Check sheet for the drawn part. Datum: minimum x, y, z corner. Units: mm. A direction names the side the tool comes from. Coordinates: 2 decimals unless noted, no trailing zeros. Write each loop counter-clockwise with the first axis right and the second up, starting at its lowest first coordinate (ties: lowest second). Pieces come first, ordered by that corner, then holes. Notation, with made-up numbers: (17, 17.25) -> (34, 17.25) arc R7 ccw to (34, 25.25) -> close; hole circle Ø4 at (38, -15). An arc over 180 degrees is marked (long way). Answer in a Markdown table with one row per item.
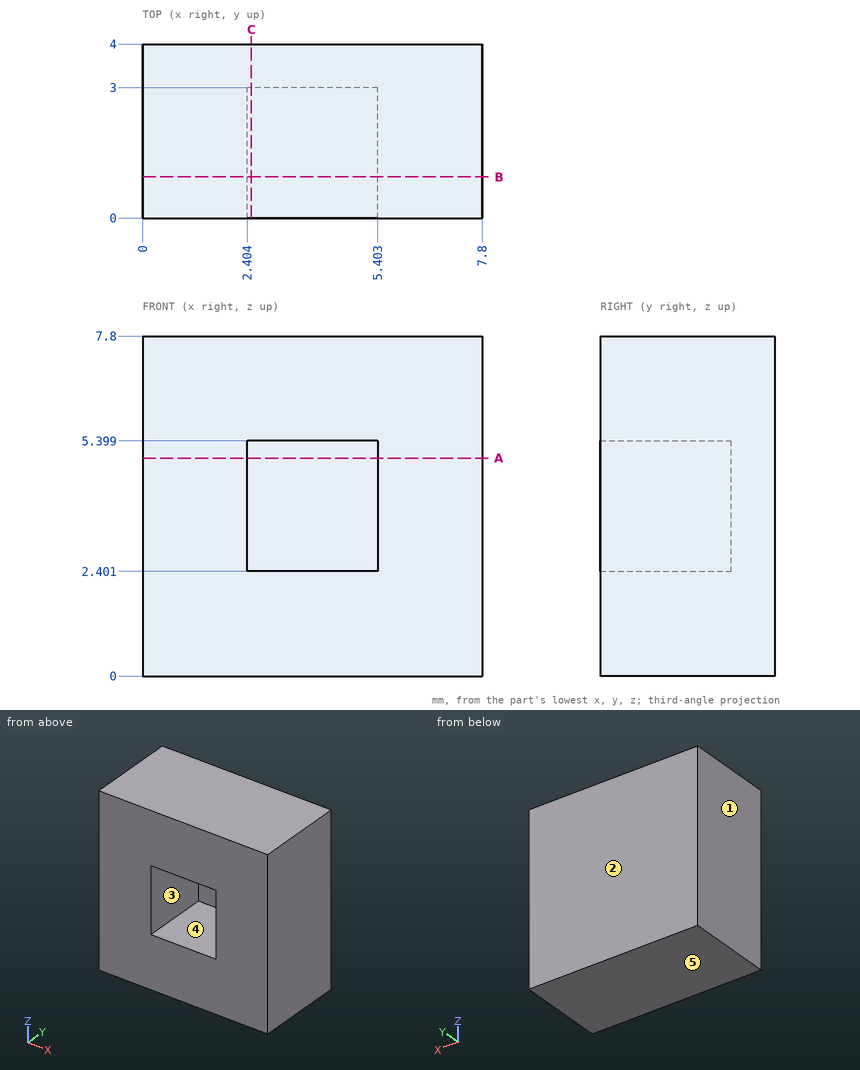
1. Release check for a two-part mould opening along X. For the marked faces 1, 2 and 3 record: released by +X, released by -X, zero draft, split by the parting line, or undercut.
Findings below:
| item | result |
|---|---|
| face 1 | released by -X |
| face 2 | zero draft |
| face 3 | undercut |
2. Sectioned sample at A-A, the plane z = 5. Record the cut outline in (x, y) (1 decimal), and give its area (3 significant figures).
Findings below:
| item | result |
|---|---|
| outline | (0, 0) -> (2.4, 0) -> (2.4, 3) -> (5.4, 3) -> (5.4, 0) -> (7.8, 0) -> (7.8, 4) -> (0, 4) -> close |
| area | 22.2 mm² |
3. Material ranges on probe 1 along X at (y, z) = (1.85, 4.75) (1 decimal); probe 2 along Y at (x, z) = (3, 2.5), recorded low to high. Write a range as from..to.
Findings below:
| item | result |
|---|---|
| probe 1 | x = 0..2.4, 5.4..7.8 |
| probe 2 | y = 3..4 |
4. Sectioned sample at C-C, the plane x = 2.5. Record the cut outline in (y, z), and give its area (3 significant figures).
Findings below:
| item | result |
|---|---|
| outline | (0, 0) -> (4, 0) -> (4, 7.8) -> (0, 7.8) -> (0, 5.4) -> (3, 5.4) -> (3, 2.4) -> (0, 2.4) -> close |
| area | 22.2 mm² |
5. Access from +Z, -Z, +X, -X, +Y, -Y to the whole of each face (thin tool, end or side, straight path). Record for the marked faces 4 and 5.
Findings below:
| item | result |
|---|---|
| face 4 | -Y |
| face 5 | -Z, +X, -X, +Y, -Y |
6. Sectioned sample at B-B, the plane y = 0.95. Record the cut outline in (x, z) (1 decimal).
Findings below:
| item | result |
|---|---|
| outline | (0, 0) -> (7.8, 0) -> (7.8, 7.8) -> (0, 7.8) -> close; hole (2.4, 2.4) -> (5.4, 2.4) -> (5.4, 5.4) -> (2.4, 5.4) -> close |
7. Go/stop test with flat-tipped pins: pin 1 (1.5 mm diameter, centred on x = 3.5, z = 4, fed in from -Y); pin 2 (1 mm diameter, centred on x = 5, y = 1.5, fed in from -Z). Record where each tip stops, or that it passes through.
Findings below:
| item | result |
|---|---|
| pin 1 | stops at y = 3 |
| pin 2 | stops at z = 0 |
